from build123d import *

# Parameters (mm, degrees)
RADYUS1_R = 1
RADYUS2_R = 2


with BuildPart() as part:
    # Çizim1 → Döndür1 (revolve)
    with BuildSketch(Plane.XY, mode=Mode.PRIVATE) as d_nd_r1_sk:
        Polygon((-235, 0), (-235, 7.5), (-231, 7.5), (-231, 10), (231, 10), (231, 7.5), (235, 7.5), (235, 0), align=None)
    revolve(d_nd_r1_sk.sketch.rotate(Axis((-235, 0, 0), (1, 0, 0)), 180), axis=Axis((-235, 0, 0), (1, 0, 0)))

    # Radyus1
    radyus1_edges = [part.edges().sort_by_distance(p)[0] for p in [
        (231, 10, 0),
        (-231, 10, 0),
    ]]
    fillet(radyus1_edges, radius=RADYUS1_R)

    # Radyus2
    radyus2_edges = [part.edges().sort_by_distance(p)[0] for p in [
        (235, 7.5, 0),
        (-235, 7.5, 0),
    ]]
    fillet(radyus2_edges, radius=RADYUS2_R)


solid = part.part
Design review of the part built by this model. Coordinates are the model's own, in mm. A direction names the side the tool comes from. Give positions to 0.01 mm unless a question says otherwise; leave off trailing zeros. Order: outer loops, then holes, each group sorted by start corner. A loop starts at its lowest first (then second) coordinate and runs counter-clockwise, first axis right, second up. Notation, with made-up numbers: (-7.5, -10) - (43.5, -10) arc R27 cw to (43.5, 23) - close; hole circle Ø6 at (66, 36.5). An arc over 180 degrees is marked (long way). Use CSV: the item, a comma, the result in double quotes. Start each with the question number.
Q1. For P1, Ø4, axis at x = 154.5, z = 3.5, coming from the +Y side; P2, Ø2, axis at y = -7.5, z = -3, coming from the +X side; P3, Ø4, axis at x = -149, y = -3, coming from the -Z side, all flat-tipped, find the tip position at first contact; note any pin that passes through.
Q2. Take a section at A-A (x = -197). State the section outline as (y, z) points, and give its area (3 significant figures).
Q3. Machinability: for faces 1 (the face through (232.014, -4.032, -6.324)), 2 (the face through (235, 0, 0)), 3 (the face through (-231, -2, -7.4)), which of the approach directions +Z, -Z, +X, -X, +Y, -Y give a long, thin tool a straight path to every point of the face, cutting with its end or side? Answer none if there is none.
Q4. Draft analysis for pull direction X (two halves, no side actions). For faces 4 (the face through (-231.986, -4.032, -6.324)), 5 (the face through (231, 2, -7.4)), 6 (the face through (-235, 0, 0)), state which applies: pulls with the +X half, pulls with the -X half, needs draft (parallel to the pull), parting line crosses it, or undercut.
Q5. For line 1 (Z direction, x = -214, y = -1); line 2 (X direction, y = -7.25, z = -5.75); line 3 (Z direction, x = 56, y = -0.25), list the stretches that pass through material, from the lowest coordinate up.
Calculated:
1,P1,"stops at y = 9.89"
1,P2,"stops at x = 234.23"
1,P3,"stops at z = -9.95"
2,outline,"circle Ø20 at (0, 0)"
2,area,"314 mm²"
3,face 1,"+X"
3,face 2,"+Z, -Z, +X, +Y, -Y"
3,face 3,"-X"
4,face 4,"needs draft"
4,face 5,"pulls with the +X half"
4,face 6,"pulls with the -X half"
5,line 1,"z = -9.95 to 9.95"
5,line 2,"x = -230.97 to 230.97"
5,line 3,"z = -10 to 10"
